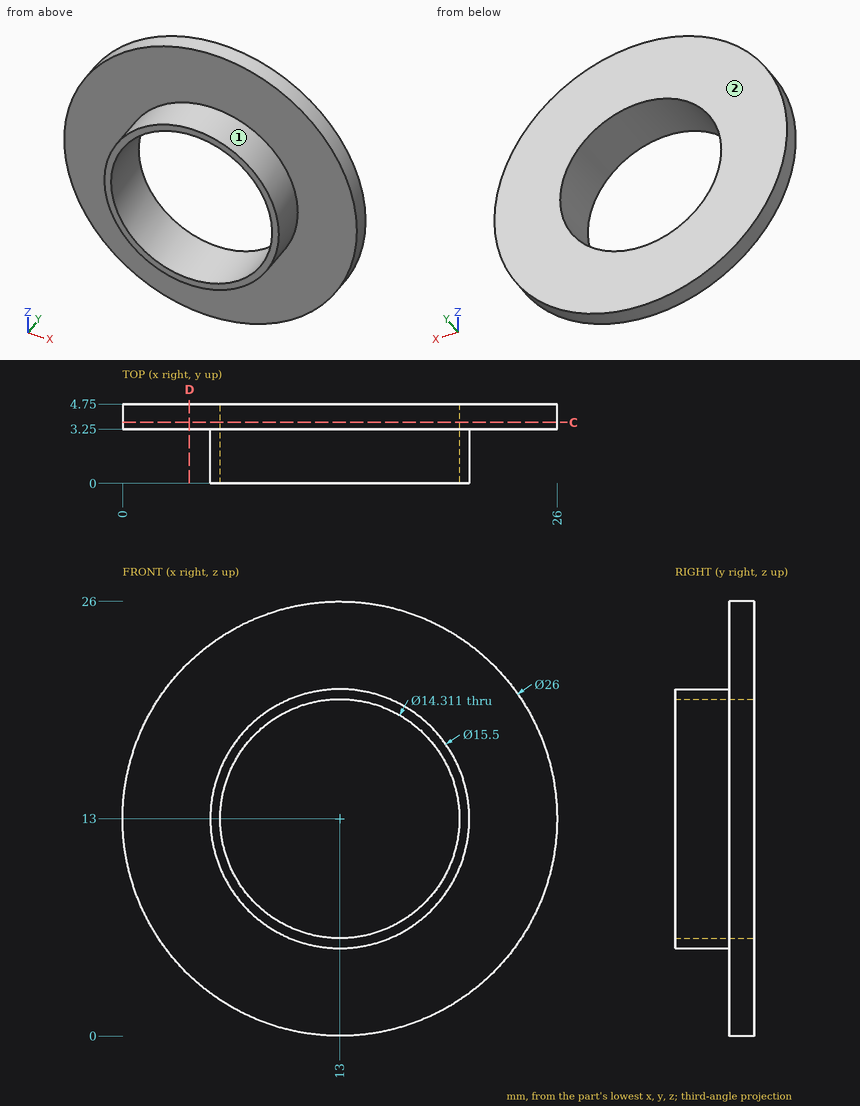
Design review of the part shown in the three views and the two pictorial views. Dimensions are in mm from the part's minimum x, y and z. A direction names the side the tool comes from. Round coordinates to 2 decimals unless told otherwise and drop trailing zeros. Write each loop counter-clockwise with the first axis right and the second up, starting at its lowest first coordinate (ties: lowest second). Pieces come first, ordered by that corner, then holes.
Item 1: Wall thickness on L1, parallel to X at y = 3.7, z = 13 (1 decimal); L2, parallel to Y at x = 17.5, z = 1.5: over which ranges is each line inside the solid? List them lowest first.
Item 2: Consider section D-D on x = 4. Give the boundary of the cut face in (y, z).
Item 3: For the marked faces 1 and 2, list the 3-axis set-ups (+Z, -Z, +X, -X, +Y, -Y) from which the entire face can be reached by the end or side of a thin tool; tool diameter is ignored.
Item 4: For pin 1 Ø1 at (x, y) = (20, 2.5) entering from -Z; pin 2 Ø3 at (x, z) = (3.5, 18.5) entering from -Y; pin 3 Ø1 at (y, z) = (2.5, 3) entering from -X, all flat-tipped, find the tip position at first contact; note any pin that passes through.
Item 5: Consider section C-C on y = 3.65. Give the boundary of the cut face in (x, z) (1 decimal), and give its area (3 significant figures).
Check values:
1. L1: x = 0 to 5.8, 20.2 to 26
1. L2: y = 3.25 to 4.75
2. outline: (3.25, 3.62) - (4.75, 3.62) - (4.75, 22.38) - (3.25, 22.38) - close
3. face 1: -Y
3. face 2: +Z, -Z, +X, -X, +Y
4. pin 1: stops at z = 8.78
4. pin 2: stops at y = 3.25
4. pin 3: passes through
5. outline: circle Ø26 at (13, 13); hole circle Ø14.3 at (13, 13)
5. area: 370 mm2
